Verification items for this drawing (mm, ordinates from the low corner). Give positions to 0.01 mm unless a question says otherwise; leave off trailing zeros. Loops run counter-clockwise (first coordinate to the right, second up) from the corner with the lowest first, then second, coordinate; pieces in that order, holes last. Notation, with made-up numbers: (54.5, 43.5) -> (67.5, 43.5) arc R20 ccw to (67.5, 73.5) -> close; hole circle Ø11 at (-25, 72). An arc over 180 degrees is marked (long way). Answer as CSV lines item,"result". Start each with the question number.
(1) Release check for a two-part mould opening along Z. For the marked faces 1, 2, 3 and 4 record: pulls with the +Z half, pulls with the -Z half, needs draft (parallel to the pull), parting line crosses it, or undercut.
(2) Section check A-A on z = 34. Enter the section's corners in (x, y) (1 decimal), plus the area to 3 significant figures.
(3) Gauge pin test, flat ends, axial feed: pin 1 Ø5 at (x, y) = (28.5, 40) entering from -Z; pin 2 Ø1.2 at (y, z) = (58, 60) entering from +X (3 decimals); pin 3 Ø7 at (x, y) = (111, 72.5) entering from +Z. Record the tip position at first contact, or that the pin passes through.
(4) Section check D-D on x = 104.5. Enter the section's corners in (y, z), plus the area to 3 significant figures.
(5) Section check B-B on x = 55.5. Enter the section's corners in (y, z).
(6) Material ranges on line 1 (X direction, y = 7, z = 23) (1 decimal); line 2 (X direction, y = 8, z = 33) (1 decimal); line 3 (Z direction, x = 104, y = 67), recorded low to high. Write a range as from..to.
(7) Section check C-C on y = 81. Enter the section's corners in (x, z) (1 decimal).
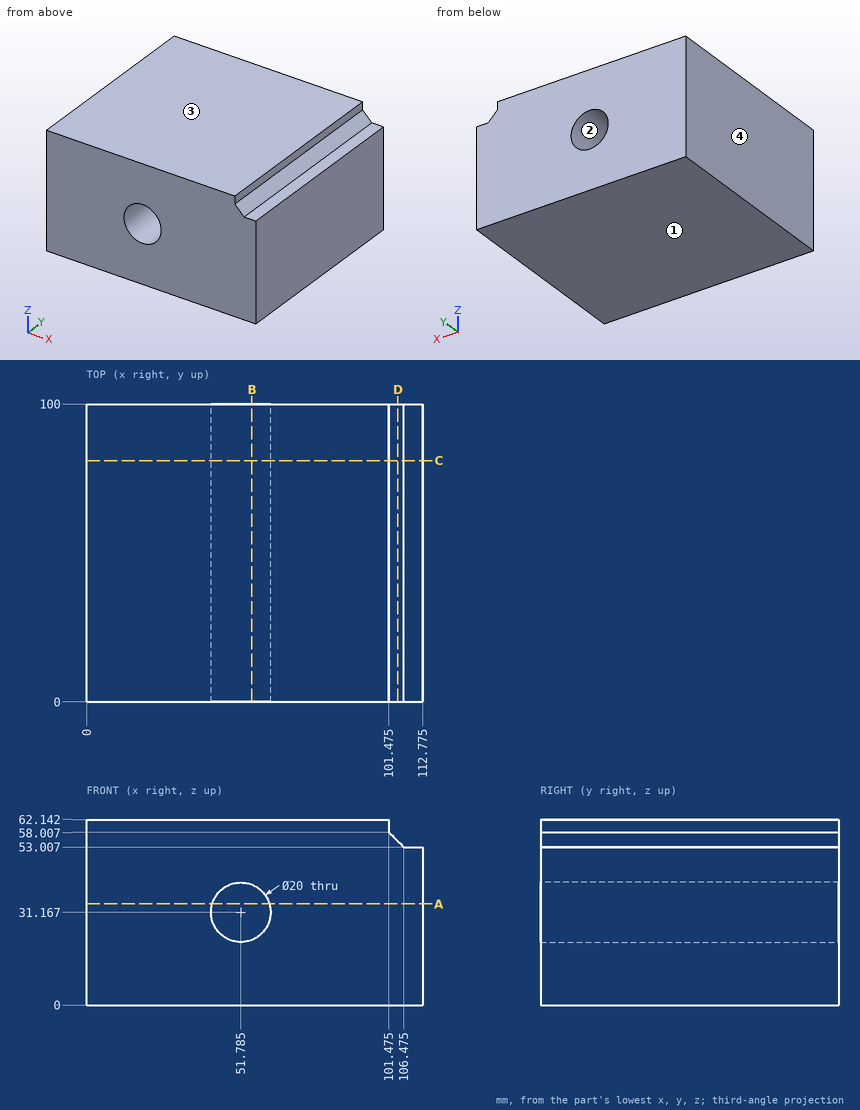
Working result:
1,face 1,"pulls with the -Z half"
1,face 2,"undercut"
1,face 3,"pulls with the +Z half"
1,face 4,"needs draft"
2,outline,"(0, 0) -> (42.2, 0) -> (42.2, 100) -> (0, 100) -> close; (61.4, 0) -> (112.8, 0) -> (112.8, 100) -> (61.4, 100) -> close"
2,area,"9,360 mm^2"
3,pin 1,"stops at z = 0"
3,pin 2,"stops at x = 101.475"
3,pin 3,"stops at z = 53.01"
4,outline,"(0, 0) -> (100, 0) -> (100, 54.98) -> (0, 54.98) -> close"
4,area,"5,500 mm^2"
5,outline,"(0, 0) -> (100, 0) -> (100, 21.88) -> (0, 21.88) -> close; (0, 40.45) -> (100, 40.45) -> (100, 62.14) -> (0, 62.14) -> close"
6,line 1,"x = 0..46, 57.6..112.8"
6,line 2,"x = 0..42, 61.6..112.8"
6,line 3,"z = 0..55.48"
7,outline,"(0, 0) -> (112.8, 0) -> (112.8, 53) -> (106.5, 53) -> (101.5, 58) -> (101.5, 62.1) -> (0, 62.1) -> close; hole circle Ø20 at (51.8, 31.2)"
